from build123d import *

# Parameters (mm, degrees)
F0_W      = 25.4
F0_H      = 25.4
F1_DEPTH  = 6.35
F2_W      = 12.7
F2_H      = 1.5875
F3_DEPTH  = 25.401
F4_W      = 12.7
F4_H      = 1.5875
F5_DEPTH  = 25.401
F6_W      = 3.5
F6_H      = 15
F6_W_2    = 3.2
F7_DEPTH  = 18
F8_R      = 7.49999
F9_R      = 5.08
F10_R     = 7
F11_DEPTH = 2
F12_D     = 5
F13_R     = 0.508
F14_R     = 0.254


# Not quite as in the source:
# - a fillet or chamfer is up to 0.001 mm smaller than in the source, because OpenCascade refuses the exact size


with BuildPart() as f1:
    # F0 (on Top) → F1 (new body)
    with BuildSketch(Plane.XY):
        Rectangle(F0_W, F0_H)
    extrude(amount=F1_DEPTH)

    # F2 (on face) → F3 (cut, through all)
    with BuildSketch(Plane.YZ.offset(12.7)):
        with Locations((0, 2.38125)):
            Rectangle(F2_W, F2_H)
    extrude(amount=-F3_DEPTH, mode=Mode.SUBTRACT)

    # F4 (on face) → F5 (cut, through all)
    with BuildSketch(Plane.XZ.offset(12.7)):
        with Locations((0, 3.96875)):
            Rectangle(F4_W, F4_H)
    extrude(amount=-F5_DEPTH, mode=Mode.SUBTRACT)

    # F6 (on face) → F7 (join)
    with BuildSketch(Plane.XY.offset(6.35)):
        with Locations((-6.35, 0)):
            Rectangle(F6_W, F6_H)
        Rectangle(F6_W_2, F6_H)
        with Locations((6.35, 0)):
            Rectangle(F6_W, F6_H)
    extrude(amount=F7_DEPTH)

    # F8 (radius 7.5 in the source; OpenCascade refuses exactly that, so slightly less here)
    f8_edges = [f1.edges().sort_by_distance(p)[0] for p in [
        (6.35, -7.5, 24.35),
        (0, -7.5, 24.35),
        (-6.35, -7.5, 24.35),
        (-6.35, 7.5, 24.35),
        (6.35, 7.5, 24.35),
        (0, 7.5, 24.35),
    ]]
    fillet(f8_edges, radius=F8_R)

    # F9
    f9_edges = [f1.edges().sort_by_distance(p)[0] for p in [
        (12.7, 12.7, 3.175),
        (12.7, -12.7, 3.175),
        (-12.7, 12.7, 3.175),
        (-12.7, -12.7, 3.175),
    ]]
    fillet(f9_edges, radius=F9_R)

    # F10 (on face) → F11 (join)
    with BuildSketch(Plane.YZ.offset(8.1)):
        with Locations((0, 16.85)):
            Circle(F10_R)
        Polygon((-4.5135996016, 15.6263094195), (-3.3165469299, 20.1470466272), (1.1970526717, 21.3707372077), (4.5135996016, 18.0736905805), (3.3165469299, 13.5529533728), (-1.1970526717, 12.3292627923), align=None, mode=Mode.SUBTRACT)
    extrude(amount=F11_DEPTH)

    # F12 (through all)
    with Locations(Plane.YZ.offset(8.1)):
        with Locations((0, 16.85)):
            Hole(F12_D / 2)

    # F13
    f13_edges = [f1.edges().sort_by_distance(p)[0] for p in [
        (10.1, -7, 16.85),
    ]]
    fillet(f13_edges, radius=F13_R)

    # F14
    f14_edges = [f1.edges().sort_by_distance(p)[0] for p in [
        (-12.7, 0, 1.5875),
        (0, -12.7, 3.175),
        (12.7, 0, 1.5875),
        (0, 12.7, 3.175),
    ]]
    fillet(f14_edges, radius=F14_R)


solid = f1.part
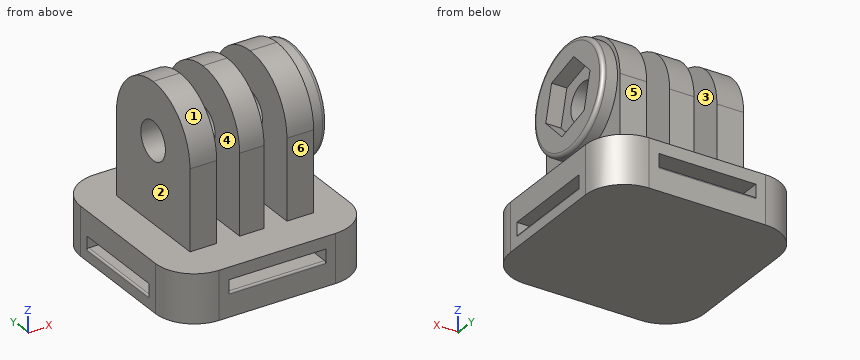
CAD build for the part. Positions are in the model's coordinates, mm. Face numbers are marked on the shaded views. A direction names the side the tool comes from. Coordinates: 2 decimals unless noted, no trailing zeros. Write each loop counter-clockwise with the first axis right and the second up, starting at its lowest first coordinate (ties: lowest second). Pieces come first, ordered by that corner, then holes. Notation, with made-up numbers: M 50.5,83.5 L 108.5,83.5 A16 cw 108.5,98.5 Z; hole C -34.75,53.25 d1. An arc over 180 degrees is marked long. Return JSON: item names as keys, results as strings.
Item 1: Which spindle directions (+Z, -Z, +X, -X, +Y, -Y) get a long thin tool onto all of the face, cutting with end or side? Do the marked faces 4, 5 and 6. Say none if no direction does.
Findings below:
{"face 4": "+Z, +Y, -Y", "face 5": "+Z, +X, -X, +Y", "face 6": "+Z, +X, -X, -Y"}
Item 2: Two-plate mould, pull along X, no slides. Class the marked faces 1, 2 and 3: +X half, -X half, draft (parallel to the pull), parting line (faces both ways), or undercut.
Findings below:
{"face 1": "draft", "face 2": "-X half", "face 3": "undercut"}
Item 3: Slice it at A-A, the plane z = 4. Write the cut outline in (x, y).
Findings below:
{"outline": "M -12.7,-7.62 A5.08 ccw -7.62,-12.7 L -6.35,-12.7 L -6.35,12.7 L -7.62,12.7 A5.08 ccw -12.7,7.62 Z; M 6.35,-12.7 L 7.62,-12.7 A5.08 ccw 12.7,-7.62 L 12.7,7.62 A5.08 ccw 7.62,12.7 L 6.35,12.7 Z"}
Item 4: Drop flat-ended pins along their axis: pin 1 Ø3 at (y, z) = (0, 16.85) entering from +X; pin 2 Ø1.6 at (x, z) = (0.5, 11) entering from +Y; pin 3 Ø1 at (x, z) = (-6.5, 21.5) entering from +Y; pin 4 Ø8 at (y, z) = (0, 16.85) entering from +X. Give the stop position or say it passes through.
Findings below:
{"pin 1": "passes through", "pin 2": "stops at y = 7.5", "pin 3": "stops at y = 6.25", "pin 4": "stops at x = 8.1"}
Item 5: Probe line 1 (X direction, y = 6.75, z = 7.25); line 2 (Z direction, x = -0.8, y = 0); line 3 (X direction, y = 6, z = 14.5). List the from-to ranges inside material, lowest first. Write a range as from..to.
Findings below:
{"line 1": "x = -8.1..-4.6, -1.6..1.6, 4.6..8.1", "line 2": "z = 0..1.59, 4.76..14.35, 19.35..24.35", "line 3": "x = -8.1..-4.6, -1.6..1.6, 4.6..10.1"}
Item 6: Slice it at D-D, the plane x = 8.75. State how many separate pieces and enclosed holes the cut face has, and give its area (3 significant figures).
Findings below:
{"separate pieces": "2", "enclosed holes": "2", "area": "237 mm2"}
